from build123d import *

# Parameters (mm, degrees)
SKETCH1_R                  = 15.875
SKETCH1_R_2                = 4.7625
BOSS_EXTRUDE1_DEPTH        = 4.7625
F_10_CLEARANCE_HOLE1_D     = 4.9784
LPATTERN1_COUNT            = 4
LPATTERN1_PITCH            = 80
CUT_EXTRUDE1_DEPTH         = 10
FILLET1_R                  = 4
CUT_EXTRUDE2_DEPTH         = 5.7625
FILLET2_R                  = 4
LPATTERN2_COUNT            = 4
LPATTERN2_PITCH            = 80
FILLET1_OF_LPATTERN2_R     = 4
LPATTERN3_COUNT            = 3
LPATTERN3_PITCH            = 80
FILLET2_OF_LPATTERN3_R     = 4
LPATTERN4_COUNT            = 2
LPATTERN4_PITCH            = 80
FILLET2_OF_LPATTERN4_R     = 4
LPATTERN5_COUNT            = 2
LPATTERN5_PITCH            = 80
FILLET1_OF_LPATTERN5_R     = 4
F_10_CLEARANCE_HOLE2_D     = 4.9784
F_10_CLEARANCE_HOLE2_DEPTH = 4.7625


with BuildPart() as part:
    # Sketch1 → Boss-Extrude1 (new body)
    with BuildSketch(Plane.XY):
        with BuildLine():
            Line((-212.5, 35), (212.5, 35))
            Line((212.5, 35), (212.5, -35))
            Line((212.5, -35), (-212.5, -35))
            ThreePointArc((-212.5, -35), (-216.530381946, -34.767168728), (-220.507141095, -34.07177265))
            Line((-220.507141095, -34.07177265), (-314.360273, -12.015530461))
            ThreePointArc((-314.360273, -12.015530461), (-325.748634462, 2.719438205), (-313.666145568, 16.890801601))
            Line((-313.666145568, 16.890801601), (-218.862525007, 34.416831283))
            ThreePointArc((-218.862525007, 34.416831283), (-215.694597401, 34.853902901), (-212.5, 35))
        make_face()
        with Locations((-212.5, 0)):
            Circle(SKETCH1_R, mode=Mode.SUBTRACT)
        with Locations((-310.980775301, 2.364817767)):
            Circle(SKETCH1_R_2, mode=Mode.SUBTRACT)
    extrude(amount=BOSS_EXTRUDE1_DEPTH)

    # #10 Clearance Hole1 (through all)
    with Locations(Plane(origin=(0, 0, 0), x_dir=(-1, 0, 0), z_dir=(0, 0, -1))):
        with Locations((-126.15, 25), (-86.15, -25)):
            f_10_clearance_hole1 = Hole(F_10_CLEARANCE_HOLE1_D / 2)

    # LPattern1: #10 Clearance Hole1 ×4
    with Locations(*[(-i * LPATTERN1_PITCH, 0, 0) for i in range(1, LPATTERN1_COUNT)]):
        add(f_10_clearance_hole1, mode=Mode.SUBTRACT)

    # Sketch13 → Cut-Extrude1 (cut)
    with BuildSketch(Plane(origin=(0, 0, 0), x_dir=(-1, 0, 0), z_dir=(0, 0, -1))):
        Polygon((-56.301294523, 22.715958732), (-86.15, -14.594923114), (-115.998705477, 22.715958732), align=None)
    cut_extrude1 = extrude(amount=-CUT_EXTRUDE1_DEPTH, mode=Mode.SUBTRACT)

    # Fillet1
    fillet1_edges = [part.edges().sort_by_distance(p)[0] for p in [
        (56.301294523, 22.715958732, 2.38125),
        (86.15, -14.594923114, 2.38125),
        (115.998705477, 22.715958732, 2.38125),
    ]]
    fillet(fillet1_edges, radius=FILLET1_R)

    # Sketch14 → Cut-Extrude2 (cut, through all)
    with BuildSketch(Plane(origin=(0, 0, 0), x_dir=(-1, 0, 0), z_dir=(0, 0, -1))):
        Polygon((-46.15, 14.594923114), (-75.998705477, -22.715958732), (-16.301294523, -22.715958732), align=None)
    cut_extrude2 = extrude(amount=-CUT_EXTRUDE2_DEPTH, mode=Mode.SUBTRACT)

    # Fillet2
    fillet2_edges = [part.edges().sort_by_distance(p)[0] for p in [
        (46.15, 14.594923114, 2.38125),
        (16.301294523, -22.715958732, 2.38125),
        (75.998705477, -22.715958732, 2.38125),
    ]]
    fillet(fillet2_edges, radius=FILLET2_R)

    # LPattern2: Cut-Extrude1 ×4
    with Locations(*[(-i * LPATTERN2_PITCH, 0, 0) for i in range(1, LPATTERN2_COUNT)]):
        add(cut_extrude1, mode=Mode.SUBTRACT)

    # Fillet1 of LPattern2
    fillet1_of_lpattern2_edges = [part.edges().sort_by_distance(p)[0] for p in [
        (-23.698705477, 22.715958732, 2.38125),
        (6.15, -14.594923114, 2.38125),
        (35.998705477, 22.715958732, 2.38125),
        (-103.698705477, 22.715958732, 2.38125),
        (-73.85, -14.594923114, 2.38125),
        (-44.001294523, 22.715958732, 2.38125),
        (-183.698705477, 22.715958732, 2.38125),
        (-153.85, -14.594923114, 2.38125),
        (-124.001294523, 22.715958732, 2.38125),
    ]]
    fillet(fillet1_of_lpattern2_edges, radius=FILLET1_OF_LPATTERN2_R)

    # LPattern3: Cut-Extrude2 ×3
    with Locations(*[(-i * LPATTERN3_PITCH, 0, 0) for i in range(1, LPATTERN3_COUNT)]):
        add(cut_extrude2, mode=Mode.SUBTRACT)

    # Fillet2 of LPattern3
    fillet2_of_lpattern3_edges = [part.edges().sort_by_distance(p)[0] for p in [
        (-33.85, 14.594923114, 2.38125),
        (-63.698705477, -22.715958732, 2.38125),
        (-4.001294523, -22.715958732, 2.38125),
        (-113.85, 14.594923114, 2.38125),
        (-143.698705477, -22.715958732, 2.38125),
        (-84.001294523, -22.715958732, 2.38125),
    ]]
    fillet(fillet2_of_lpattern3_edges, radius=FILLET2_OF_LPATTERN3_R)

    # LPattern4: Cut-Extrude2 ×2
    with Locations(*[(i * LPATTERN4_PITCH, 0, 0) for i in range(1, LPATTERN4_COUNT)]):
        add(cut_extrude2, mode=Mode.SUBTRACT)

    # Fillet2 of LPattern4
    fillet2_of_lpattern4_edges = [part.edges().sort_by_distance(p)[0] for p in [
        (126.15, 14.594923114, 2.38125),
        (96.301294523, -22.715958732, 2.38125),
        (155.998705477, -22.715958732, 2.38125),
    ]]
    fillet(fillet2_of_lpattern4_edges, radius=FILLET2_OF_LPATTERN4_R)

    # LPattern5: Cut-Extrude1 ×2
    with Locations(*[(i * LPATTERN5_PITCH, 0, 0) for i in range(1, LPATTERN5_COUNT)]):
        add(cut_extrude1, mode=Mode.SUBTRACT)

    # Fillet1 of LPattern5
    fillet1_of_lpattern5_edges = [part.edges().sort_by_distance(p)[0] for p in [
        (136.301294523, 22.715958732, 2.38125),
        (166.15, -14.594923114, 2.38125),
        (195.998705477, 22.715958732, 2.38125),
    ]]
    fillet(fillet1_of_lpattern5_edges, radius=FILLET1_OF_LPATTERN5_R)

    # #10 Clearance Hole2
    with Locations(Plane.XY.offset(4.7625)):
        with Locations((206.15, 25), (206.15, -25), (166.15, -25)):
            Hole(F_10_CLEARANCE_HOLE2_D / 2, depth=F_10_CLEARANCE_HOLE2_DEPTH)


solid = part.part
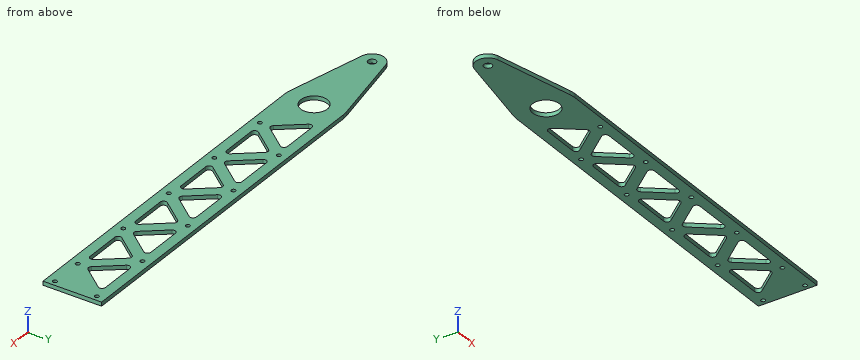
Source: CAD feature listing. Evaluate the final solid. Frame: model axes, mm. Round coordinates to 2 decimals unless told otherwise and drop trailing zeros. Order: outer loops, then holes, each group sorted by start corner. A loop starts at its lowest first (then second) coordinate and runs counter-clockwise, first axis right, second up. Notation, with made-up numbers: (20.5, 50) -> (63.5, 50) arc R16 cw to (63.5, 55) -> close; hole circle Ø10 at (80, 57.25). An arc over 180 degrees is marked (long way). Answer as CSV lines item,"result".
Item 1: Line query: L1, parallel to Y at x = 206.15, z = 3.6; L2, parallel to Y at x = -73.85, z = 1.65; L3, parallel to Y at x = 54, z = 0.65. Output: solid intervals per line, ascending.
A:
L1,"-35 to -27.49, -22.51 to 22.51, 27.49 to 35"
L2,"-35 to -27.49, -22.51 to -12.19, 22.72 to 35"
L3,"-35 to -22.72, 4.78 to 35"
Item 2: Section B-B, the plane x = -291. Return loops of the section in (y, z), plus the area to 3 significant figures.
A:
outline,"(-17.51, 0) -> (21.08, 0) -> (21.08, 4.76) -> (-17.51, 4.76) -> close"
area,"184 mm²"
Item 3: Section A-A, the plane z = 1.8. Count the separate pieces of the cut face and the enclosed holes in it, plus the area to 3 significant figures.
A:
separate pieces,"1"
enclosed holes,"22"
area,"24,300 mm²"
